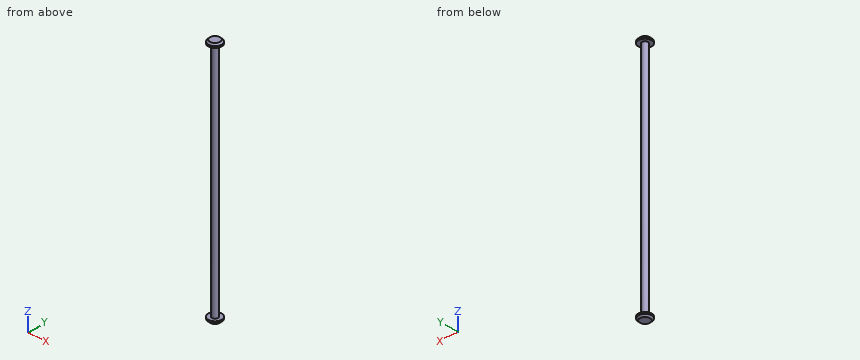
```python
from build123d import *

# Parameters (mm, degrees)
SKETCH_1_R      = 0.925
EXTRUDE_1_DEPTH = 70.5
SKETCH_2_R      = 2
EXTRUDE_2_DEPTH = 1
EXTRUDE_START   = 1
SKETCH_3_R      = 2
EXTRUDE_3_DEPTH = 1
CHAMFER_1_SIZE  = 0.5
CHAMFER_2_SIZE  = 0.5


with BuildPart() as part:
    # 스케치1 → 보스-돌출1 (new body)
    with BuildSketch(Plane.XY):
        Circle(SKETCH_1_R)
    extrude(amount=EXTRUDE_1_DEPTH)

    # 스케치2 → 보스-돌출2 (add)
    with BuildSketch(Plane.XY.offset(70.5)):
        Circle(SKETCH_2_R)
    extrude(amount=EXTRUDE_2_DEPTH)

    # 스케치3 → 보스-돌출3 (add)
    with BuildSketch(Plane(origin=(0, 0, 0), x_dir=(-1, 0, 0), z_dir=(0, 0, -1)).offset(EXTRUDE_START)):
        with Locations(Location((0, 0, 0), (0, 0, 180))):
            Circle(SKETCH_3_R)
    extrude(amount=-EXTRUDE_3_DEPTH)

    # 모따기1
    chamfer_1_edges = [part.edges().sort_by_distance(p)[0] for p in [
        (-2, 0, 71.5),
    ]]
    chamfer(chamfer_1_edges, length=CHAMFER_1_SIZE)

    # 모따기2
    chamfer_2_edges = [part.edges().sort_by_distance(p)[0] for p in [
        (-2, 0, -1),
    ]]
    chamfer(chamfer_2_edges, length=CHAMFER_2_SIZE)


solid = part.part
```
The model under review builds one solid part; all positions refer to its coordinate system, in mm. Give positions to 0.01 mm unless a question says otherwise; leave off trailing zeros. Loops run counter-clockwise (first coordinate to the right, second up) from the corner with the lowest first, then second, coordinate; pieces in that order, holes last. Notation, with made-up numbers: (85, -15) - (134, -15) arc R11 cw to (134, -11) - close; hole circle Ø11 at (-3.5, 47.25). An arc over 180 degrees is marked (long way). Answer as a JSON object with one key per item and string values.
Q1. Add section A-A on x = 0. State the section outline as (y, z) points (3 decimals).
Worked out:
{"outline": "(-2, -0.5) - (-1.5, -1) - (1.5, -1) - (2, -0.5) - (2, 0) - (0.925, 0) - (0.925, 70.5) - (2, 70.5) - (2, 71) - (1.5, 71.5) - (-1.5, 71.5) - (-2, 71) - (-2, 70.5) - (-0.925, 70.5) - (-0.925, 0) - (-2, 0) - close"}
Q2. Add section C-C on z = 58.5. State the section outline as (x, y) points (3 decimals).
Worked out:
{"outline": "circle Ø1.85 at (0, 0)"}
Q3. Insertion check: pin 1 (2 mm diameter, centred on x = 1, z = 56, fed in from -Y) (3 decimals); pin 2 (1 mm diameter, centred on y = 0.5, z = 24.5, fed in from -X) (3 decimals). Each pin has a flat end and moves straight along its axis. Give the tip position at first contact, or say it passes through.
Worked out:
{"pin 1": "stops at y = -0.925", "pin 2": "stops at x = -0.925"}
Q4. To check wall thickness, follow line 1 along Z through (x, y) = (-0.7, -0.7); line 2 along Z through (x, y) = (-0.9, 1.65); line 3 along X through (y, z) = (0.1, 38.5). State the ranges of each line that lie inside material, in increasing order.
Worked out:
{"line 1": "z = -1 to 0, 70.5 to 71.5", "line 2": "z = -0.62 to 0, 70.5 to 71.12", "line 3": "x = -0.92 to 0.92"}
